Verification items for the finished model (mm, model axes). A direction names the side the tool comes from. Give positions to 0.01 mm unless a question says otherwise; leave off trailing zeros. Loops run counter-clockwise (first coordinate to the right, second up) from the corner with the lowest first, then second, coordinate; pieces in that order, holes last. Notation, with made-up numbers: (57.25, 8.5) - (100.25, 8.5) arc R17 cw to (100.25, 27.5) - close; hole circle Ø11 at (1.25, 15). An arc over 180 degrees is marked (long way). One line per item, written item: value. Start each with the question number.
1. Sectioned sample at C-C (y = 15). Record the cut outline in (x, z).
2. Mould release check, pull along Y, two halves, no side actions. Record for faces 4 (the flat face through (0, 11.43, 9)), 5 (the flat face through (-7.62, 8, -3)), 6 (the flat face through (2.54, 27, -9)): pulls with the +Y half, pulls with the -Y half, needs draft (parallel to the pull), parting line crosses it, or undercut.
3. Sectioned sample at D-D (x = 9). Record the cut outline in (y, z).
4. Sectioned sample at A-A (x = 0). Record the cut outline in (y, z) (3 decimals).
5. Access from +Z, -Z, +X, -X, +Y, -Y to the whole of each face (thin tool, end or side, straight path). Record for faces 1 (the cylindrical face through (0.33, 17.23, 2.52)), 2 (the flat face through (-10, 11.43, 0)), 3 (the flat face through (0, 31.496, -8)).
6. Scan lines: L1, parallel to X at y = 5, z = -11.5; L2, parallel to Y at x = -1, z = -11.25; L3, parallel to Y at x = 4.4, z = 0 (3 decimals). Record each from-to range of solid material in increasing order. Write a range as [from, to].
7. Sectioned sample at B-B (y = 5.08). Record the cut outline in (x, z) (3 decimals).
8. Gauge pin test, flat ends, axial feed: pin 1 (5 mm diameter, centred on y = 5.08, z = 0, fed in from +X); pin 2 (1 mm diameter, centred on x = 5.5, z = -7, fed in from +Y); pin 3 (1 mm diameter, centred on x = -6.5, y = 7.5, fed in from -Z); pin 4 (3 mm diameter, centred on y = 28.5, z = 11, fed in from -X). Record the tip position at first contact, or that the pin passes through.
from build123d import *

# Parameters (mm, degrees)
CUT_EXTRUDE1_DEPTH      = 11.43
SKETCH3_R               = 3.175
CUT_EXTRUDE2_DEPTH      = 50.355147776
CUT_EXTRUDE3_DEPTH      = 47.487551581
CUT_EXTRUDE3_DEPTH_BACK = 47.487551581
SKETCH4_W               = 5.08
SKETCH4_H               = 1.27
FILLET1_R               = 1.905


with BuildPart() as part:
    # Sketch1 → Revolve1 (revolve)
    with BuildSketch(Plane.XY):
        with BuildLine():
            Line((0, 0), (0, 5.602635041))
            Line((0, 5.602635041), (-2.54, 5.602635041))
            Line((-2.54, 5.602635041), (-2.54, 22.86))
            ThreePointArc((-2.54, 22.86), (-5.294384008, 28.994194932), (0, 33.139611281))
            Line((0, 33.139611281), (0, 41.91))
            ThreePointArc((0, 41.91), (-10.057886856, 37.743886856), (-14.224, 27.686))
            Line((-14.224, 27.686), (-14.224, 0))
            Line((-14.224, 0), (0, 0))
        make_face()
    revolve(axis=Axis((0, 0, 0), (0, 1, 0)))

    # Sketch2 → Cut-Extrude1 (cut)
    with BuildSketch(Plane.XZ):
        with BuildLine():
            Line((-2.54, 13.995376951), (-2.54, -13.995376951))
            ThreePointArc((-2.54, -13.995376951), (0, -14.224), (2.54, -13.995376951))
            Line((2.54, -13.995376951), (2.54, 13.995376951))
            ThreePointArc((2.54, 13.995376951), (0, 14.224), (-2.54, 13.995376951))
        make_face()
        with BuildLine():
            Line((-7.62, 12.010735864), (-7.62, -12.010735864))
            ThreePointArc((-7.62, -12.010735864), (-14.224, 0), (-7.62, 12.010735864))
        make_face()
        with BuildLine():
            Line((7.62, 12.010735864), (7.62, -12.010735864))
            ThreePointArc((7.62, -12.010735864), (14.224, 0), (7.62, 12.010735864))
        make_face()
    extrude(amount=-CUT_EXTRUDE1_DEPTH, mode=Mode.SUBTRACT)

    # Sketch3 → Cut-Extrude2 (cut, through all)
    with BuildSketch(Plane.ZY.offset(7.62)):
        with Locations((0, 5.08)):
            Circle(SKETCH3_R)
        with BuildLine():
            Line((3.510108408, 1.40773381), (13.995376951, 11.43))
            Line((13.995376951, 11.43), (13.995376951, 0))
            Line((13.995376951, 0), (0, 0))
            ThreePointArc((0, 0), (1.890937302, 0.365049722), (3.510108408, 1.40773381))
        make_face()
    extrude(amount=-CUT_EXTRUDE2_DEPTH, mode=Mode.SUBTRACT)

    # Sketch4 → Cut-Extrude3 (cut, two sides: drawn at the far end of the back side and taken through both)
    with BuildSketch(Plane.XY.offset(-CUT_EXTRUDE3_DEPTH_BACK)):
        with Locations((0, 27.051)):
            Rectangle(SKETCH4_W, SKETCH4_H)
        with Locations((0, 32.131)):
            Rectangle(SKETCH4_W, SKETCH4_H)
    extrude(amount=CUT_EXTRUDE3_DEPTH + CUT_EXTRUDE3_DEPTH_BACK, mode=Mode.SUBTRACT)

    # Fillet1
    # the kernel refuses this fillet: 1.905 mm, written as the material it takes off along each edge
    with BuildSketch(Plane(origin=(0, 27.686, 0), x_dir=(-0.5373639456593198, 0, 0.8433504549743527), z_dir=(-0.8433504549743527, 0, -0.5373639456593198))) as fillet1_piece_1_section:
        with BuildLine():
            CenterArc((12.170814928, 1.905), FILLET1_R, 270, 98.895870208)
            Line((12.170814928, 0), (14.224, 0))
            ThreePointArc((14.224, 0), (14.181160416, 1.10311616), (14.05289971, 2.199587629))
        make_face()
    fillet1_piece_1 = revolve(axis=Axis((0, 27.686, 0), (0, 1, 0)), revolution_arc=65.00874172, mode=Mode.PRIVATE)
    fillet1_piece_1 = split(fillet1_piece_1, bisect_by=Plane(origin=(2.54, 28.192059722, 13.665836287), z_dir=(-1, 0, 0)), keep=Keep.TOP, mode=Mode.PRIVATE)
    fillet1_piece_1 = split(fillet1_piece_1, bisect_by=Plane(origin=(-2.54, 28.192059722, 13.665836287), z_dir=(1, 0, 0)), keep=Keep.TOP, mode=Mode.PRIVATE)
    add(fillet1_piece_1, mode=Mode.SUBTRACT)
    with BuildSketch(Plane(origin=(0, 31.496, 0), x_dir=(0.46799048823775274, 0, 0.883733502204703), z_dir=(0.883733502204703, 0, -0.46799048823775274))) as fillet1_piece_2_section:
        with BuildLine():
            CenterArc((12.170814928, 1.905), FILLET1_R, 270, 81.104129792)
            Line((12.170814928, 0), (13.704235696, 0))
            ThreePointArc((13.704235696, 0), (13.90190629, 0.80015324), (14.05289971, 1.610412371))
        make_face()
    fillet1_piece_2 = revolve(axis=Axis((0, 31.496, 0), (0, -1, 0)), revolution_arc=55.807867303, mode=Mode.PRIVATE)
    fillet1_piece_2 = split(fillet1_piece_2, bisect_by=Plane(origin=(-2.54, 31.138166145, 13.379180575), z_dir=(1, 0, 0)), keep=Keep.TOP, mode=Mode.PRIVATE)
    fillet1_piece_2 = split(fillet1_piece_2, bisect_by=Plane(origin=(2.54, 31.138166145, 13.379180575), z_dir=(-1, 0, 0)), keep=Keep.TOP, mode=Mode.PRIVATE)
    add(fillet1_piece_2, mode=Mode.SUBTRACT)
    with BuildSketch(Plane(origin=(0, 31.496, 0), x_dir=(-0.4679904882377507, 0, -0.883733502204704), z_dir=(-0.883733502204704, 0, 0.4679904882377507))) as fillet1_piece_3_section:
        with BuildLine():
            CenterArc((12.170814928, 1.905), FILLET1_R, 270, 81.104129792)
            Line((12.170814928, 0), (13.704235696, 0))
            ThreePointArc((13.704235696, 0), (13.90190629, 0.80015324), (14.05289971, 1.610412371))
        make_face()
    fillet1_piece_3 = revolve(axis=Axis((0, 31.496, 0), (0, -1, 0)), revolution_arc=55.807867303, mode=Mode.PRIVATE)
    fillet1_piece_3 = split(fillet1_piece_3, bisect_by=Plane(origin=(-2.54, 31.138166145, -13.379180575), z_dir=(1, 0, 0)), keep=Keep.TOP, mode=Mode.PRIVATE)
    fillet1_piece_3 = split(fillet1_piece_3, bisect_by=Plane(origin=(2.54, 31.138166145, -13.379180575), z_dir=(-1, 0, 0)), keep=Keep.TOP, mode=Mode.PRIVATE)
    add(fillet1_piece_3, mode=Mode.SUBTRACT)
    with BuildSketch(Plane(origin=(0, 27.686, 0), x_dir=(0.5373639456593708, 0, -0.84335045497432), z_dir=(0.84335045497432, 0, 0.5373639456593708))) as fillet1_piece_4_section:
        with BuildLine():
            CenterArc((12.170814928, 1.905), FILLET1_R, 270, 98.895870208)
            Line((12.170814928, 0), (14.224, 0))
            ThreePointArc((14.224, 0), (14.181160416, 1.10311616), (14.05289971, 2.199587629))
        make_face()
    fillet1_piece_4 = revolve(axis=Axis((0, 27.686, 0), (0, 1, 0)), revolution_arc=65.00874172, mode=Mode.PRIVATE)
    fillet1_piece_4 = split(fillet1_piece_4, bisect_by=Plane(origin=(-2.54, 28.192059722, -13.665836287), z_dir=(1, 0, 0)), keep=Keep.TOP, mode=Mode.PRIVATE)
    fillet1_piece_4 = split(fillet1_piece_4, bisect_by=Plane(origin=(2.54, 28.192059722, -13.665836287), z_dir=(-1, 0, 0)), keep=Keep.TOP, mode=Mode.PRIVATE)
    add(fillet1_piece_4, mode=Mode.SUBTRACT)


solid = part.part
Results are:
1. outline: circle Ø28.45 at (0, 0); hole circle Ø5.08 at (0, 0)
2. face 4: pulls with the -Y half
2. face 5: needs draft
2. face 6: undercut
3. outline: (11.43, -11.01) - (27.69, -11.01) arc R11.01 ccw to (27.69, 11.01) - (11.43, 11.01) - close
4. outline: (11.43, -14.224) - (26.416, -14.224) - (26.416, -5.304) arc R5.454 cw to (22.86, -2.54) - (11.43, -2.54) - close; (11.43, 2.54) - (22.86, 2.54) arc R5.454 cw to (26.416, 5.304) - (26.416, 14.224) - (11.43, 14.224) - close; (27.686, -12.171) arc R1.905 ccw to (31.496, -12.171) - (31.496, -3.902) arc R5.454 cw to (27.686, -5.454) - close; (27.686, 5.454) arc R5.454 cw to (31.496, 3.902) - (31.496, 12.171) arc R1.905 ccw to (27.686, 12.171) - close; (32.766, -13.286) arc R14.224 ccw to (32.766, 13.286) - (32.766, 1.984) arc R5.454 cw to (32.766, -1.984) - close
5. face 1: -Y
5. face 2: +Z, -Z, -X, -Y
5. face 3: +Z, -Z
6. L1: x = [-7.62, -2.54], [2.54, 7.62]
6. L2: y = [11.43, 26.42], [27.69, 31.5], [32.77, 36.33]
6. L3: y = [0, 1.905], [8.255, 24.464], [30.908, 41.212]
7. outline: (-7.62, -12.011) arc R14.224 ccw to (-2.54, -13.995) - (-2.54, -3.175) - (-7.62, -3.175) - close; (-7.62, 3.175) - (-2.54, 3.175) - (-2.54, 7.352) - (-7.62, 7.352) - close; (2.54, -13.995) arc R14.224 ccw to (7.62, -12.011) - (7.62, -3.175) - (2.54, -3.175) - close; (2.54, 3.175) - (7.62, 3.175) - (7.62, 7.352) - (2.54, 7.352) - close
8. pin 1: passes through
8. pin 2: stops at y = 39.16
8. pin 3: stops at z = -12.9
8. pin 4: stops at x = -10.56
